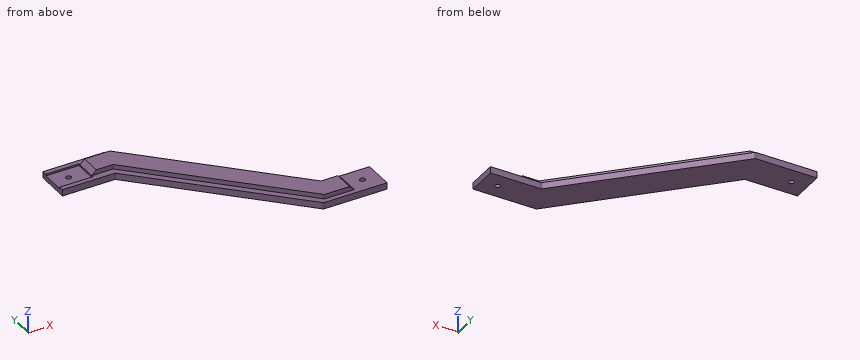
```python
from build123d import *

# Parameters (mm, degrees)
SKETCH_1_R          = 1.65
EXTRUDE_1_DEPTH     = 3
EXTRUDE_2_DEPTH     = 2.9
CHAMFER_1_SIZE      = 2.9
EXTRUDE_START       = -1.1
SKETCH_6_R          = 1.65
EXTRUDE_3_DEPTH     = 4.1
CUT_EXTRUDE_START   = 3
SKETCH_7_W          = 21
SKETCH_7_H          = 15.2
CUT_EXTRUDE_1_DEPTH = 1.1
FILLET_1_R          = 1


with BuildPart() as part:
    # 草图1 → 凸台-拉伸1 (new body)
    with BuildSketch(Plane.XY):
        Polygon((-78.55, 51.8), (-38.364971157, 51.8), (46.235028843, -32.8), (78.55, -32.8), (78.55, -51.8), (38.364971157, -51.8), (-46.235028843, 32.8), (-78.55, 32.8), align=None)
        with Locations((-68.55, 42.3)):
            Circle(SKETCH_1_R, mode=Mode.SUBTRACT)
        with Locations((68.55, -42.3)):
            Circle(SKETCH_1_R, mode=Mode.SUBTRACT)
    extrude(amount=EXTRUDE_1_DEPTH)

    # 草图2 → 凸台-拉伸2 (add)
    with BuildSketch(Plane.XY.offset(3)):
        Polygon((-57.55, 48.7), (-57.55, 35.9), (-43.950966799, 35.9), (40.649033201, -48.7), (59.55, -48.7), (59.55, -35.9), (45.950966799, -35.9), (-38.649033201, 48.7), align=None)
    extrude(amount=EXTRUDE_2_DEPTH)

    # 倒角1
    chamfer_1_edges = [part.edges().sort_by_distance(p)[0] for p in [
        (59.55, -42.3, 5.9),
        (-57.55, 42.3, 5.9),
    ]]
    chamfer(chamfer_1_edges, length=CHAMFER_1_SIZE - 0.0001)  # a hair under: the kernel refuses the full size

    # 草图6 → 凸台-拉伸3 (add)
    with BuildSketch(Plane.XY.offset(EXTRUDE_START)):
        Polygon((-78.55, 52.9), (-78.55, 31.7), (-45.135028843, 31.7), (38.364971157, -51.8), (78.55, -51.8), (78.55, -32.8), (46.235028843, -32.8), (-39.464971157, 52.9), align=None)
        with Locations((-68.55, 42.3)):
            Circle(SKETCH_6_R, mode=Mode.SUBTRACT)
        with Locations((68.55, -42.3)):
            Circle(SKETCH_6_R, mode=Mode.SUBTRACT)
    extrude(amount=EXTRUDE_3_DEPTH)

    # 草图7 → 切除-拉伸1 (cut)
    with BuildSketch(Plane.XY.offset(CUT_EXTRUDE_START)):
        with Locations((-68.05, 42.3)):
            Rectangle(SKETCH_7_W, SKETCH_7_H)
    extrude(amount=-CUT_EXTRUDE_1_DEPTH, mode=Mode.SUBTRACT)

    # 圆角1
    fillet_1_edges = [part.edges().sort_by_distance(p)[0] for p in [
        (46.235028843, -32.8, 0.95),
        (38.364971157, -51.8, 0.95),
        (-38.649033201, 48.7, 4.45),
        (-43.950966799, 35.9, 4.45),
        (40.649033201, -48.7, 4.45),
        (45.950966799, -35.9, 4.45),
        (-39.464971157, 52.9, 0.95),
        (-45.135028843, 31.7, 0.95),
    ]]
    fillet(fillet_1_edges, radius=FILLET_1_R)


solid = part.part
```
Verification items for the finished model (mm, model axes). Give positions to 0.01 mm unless a question says otherwise; leave off trailing zeros. Loops run counter-clockwise (first coordinate to the right, second up) from the corner with the lowest first, then second, coordinate; pieces in that order, holes last. Notation, with made-up numbers: M -6.5,-8.5 L 19.5,-8.5 A27 ccw 19.5,10.5 Z; hole C -33.5,72 d9. An arc over 180 degrees is marked long. Return JSON: item names as keys, results as strings.
1) Material ranges on L1, parallel to Y at x = 68.55, z = 1.15; L2, parallel to Y at x = -68.55, z = 1.15; L3, parallel to Z at x = -57, y = 34.5, recorded low to high. Write a range as [from, to].
Findings:
{"L1": "y = [-51.8, -43.95], [-40.65, -32.8]", "L2": "y = [31.7, 40.65], [43.95, 52.9]", "L3": "z = [-1.1, 3]"}
2) Section check D-D, the plane y = 7.5. Enter the section's corners in (x, z), and give its area (3 significant figures).
Findings:
{"outline": "M -20.94,-1.1 L 5.94,-1.1 L 5.94,3 L 2.55,3 L 2.55,5.9 L -15.55,5.9 L -15.55,3 L -20.94,3 Z", "area": "163 mm2"}
3) Section check B-B, the plane y = 42.3. Enter the section's corners in (x, z).
Findings:
{"outline": "M -78.55,-1.1 L -70.2,-1.1 L -70.2,1.9 L -78.55,1.9 Z; M -66.9,-1.1 L -28.86,-1.1 L -28.86,3 L -32.25,3 L -32.25,5.9 L -54.65,5.9 L -57.55,3 L -57.55,1.9 L -66.9,1.9 Z"}
4) Section check A-A, the plane x = -68.55. Enter the section's corners in (y, z), and give its area (3 significant figures).
Findings:
{"outline": "M 31.7,-1.1 L 40.65,-1.1 L 40.65,1.9 L 34.7,1.9 L 34.7,3 L 31.7,3 Z; M 43.95,-1.1 L 52.9,-1.1 L 52.9,3 L 49.9,3 L 49.9,1.9 L 43.95,1.9 Z", "area": "60.3 mm2"}
5) Section check C-C, the plane x = 68.55. Enter the section's corners in (y, z), and give its area (3 significant figures).
Findings:
{"outline": "M -51.8,-1.1 L -43.95,-1.1 L -43.95,3 L -51.8,3 Z; M -40.65,-1.1 L -32.8,-1.1 L -32.8,3 L -40.65,3 Z", "area": "64.4 mm2"}
6) Gauge pin test, flat ends, axial feed: P1, Ø3, axis at x = 68.55, y = -42.3, coming from the +Z side; P2, Ø16.5, axis at x = -64.5, y = 46, coming from the +Z side; P3, Ø0.6, axis at x = -64, z = 2.5, coming from the -Y side; P4, Ø0.6, axis at y = 44.5, z = 2.5, coming from the -X side. Record the tip position at first contact, or that the pin passes through.
Findings:
{"P1": "passes through", "P2": "stops at z = 4.3", "P3": "stops at y = 31.7", "P4": "stops at x = -57.55"}
